Source: CAD feature listing. Evaluate the final solid. Frame: model axes, mm. Face numbers are marked on the shaded views. A direction names the side the tool comes from. Round coordinates to 2 decimals unless told otherwise and drop trailing zeros. Order: outer loops, then holes, each group sorted by start corner. A loop starts at its lowest first (then second) coordinate and runs counter-clockwise, first axis right, second up. Notation, with made-up numbers: (-7.75, -2) - (23.25, -2) arc R19 ccw to (23.25, 3) - close; hole circle Ø3 at (83, 14). An arc over 180 degrees is marked (long way). Return JSON: item names as keys, results as strings. Group by question number.
1) Ray query, line 1 (X direction, y = -2, z = 8.1); line 2 (X direction, y = -6.5, z = 7.4); line 3 (Y direction, x = 8, z = 7.75). Return the intervals inside material, ascending. Write a range as from..to.
2) Mould query, pull axis Z, two halves, no side actions, for the marked faces 1, 2 and 3. Classes: pulls with the +Z half, pulls with the -Z half, needs draft (parallel to the pull), parting line crosses it, or undercut.
3) Section B-B, the plane x = 0. Return loops of the section in (y, z), plus the area to 3 significant figures.
4) Section A-A, the plane y = 0. Return loops of the section in (x, z).
5) Access query for the marked faces 4, 5 and 6. Directions: +Z, -Z, +X, -X, +Y, -Y. A direction counts if a zero-diameter tool reaches every point of the face in a straight line with its end or side. Return the directions, or none.
6) Contact query for flat-ended pins moving along their axis: P1, Ø1, axis at x = -13, z = 7.5, coming from the -Y side; P2, Ø0.6, axis at x = 17.5, z = 7.5, coming from the -Y side; P3, Ø1.3, axis at y = 0, z = 7, coming from the +X side; P4, Ø13, axis at x = -7.5, y = -3.5, coming from the +Z side. Output: stop coordinate, or through.
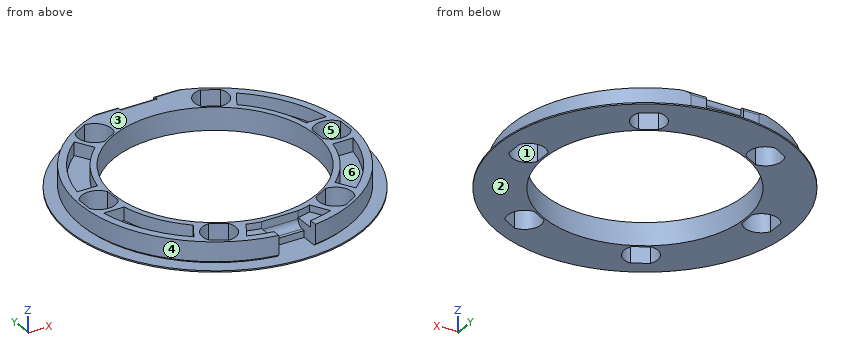
```python
from build123d import *

# Parameters (mm, degrees)
POCKET_DEPTH         = 128.037431
POLARPATTERN_COUNT   = 6
POCKET004_DEPTH      = 1.001
POCKET005_DEPTH      = 2.001
POCKET006_DEPTH      = 22.001
POCKET006_DEPTH_BACK = -22.001
POCKET007_DEPTH      = 2.75


with BuildPart() as part:
    # Sketch → Revolution (revolve)
    with BuildSketch(Plane.XZ):
        Polygon((19.85, 5.5), (22, 5.5), (22, 5.3), (15.1, 5.3), (15.1, 8.7), (20.15, 8.7), (20.15, 5.8), align=None)
    revolve(axis=Axis((0, 0, 0), (0, 0, 1)))

    # Sketch001 → Pocket (cut, through all)
    with BuildSketch(Plane.XY.offset(5.3)):
        with BuildLine():
            ThreePointArc((-15.35, 1.275735), (-17.5, 2.5), (-19.65, 1.275735))
            Line((-19.65, 1.275735), (-19.65, -1.275735))
            ThreePointArc((-19.65, -1.275735), (-17.5, -2.5), (-15.35, -1.275735))
            Line((-15.35, -1.275735), (-15.35, 1.275735))
        make_face()
    pocket = extrude(amount=POCKET_DEPTH, mode=Mode.SUBTRACT)

    # PolarPattern: Pocket ×6 about axis
    polarpattern_axis = Axis((0, 0, 0), (0, 0, 1))
    for i in range(1, POLARPATTERN_COUNT):
        add(pocket.rotate(polarpattern_axis, i * 360 / POLARPATTERN_COUNT), mode=Mode.SUBTRACT)

    # Sketch005 → Pocket004 (cut, through all)
    with BuildSketch(Plane.XY.offset(7.7)):
        with BuildLine():
            ThreePointArc((-4.775159, -15.270817), (0, -16), (4.775159, -15.270817))
            Line((4.775159, -15.270817), (6.306336, -17.922894))
            ThreePointArc((-6.306336, -17.922894), (0, -19), (6.306336, -17.922894))
            Line((-6.306336, -17.922894), (-4.775159, -15.270817))
        make_face()
    extrude(amount=POCKET004_DEPTH, mode=Mode.SUBTRACT)

    # Sketch006 → Pocket005 (cut, through all)
    with BuildSketch(Plane.XY.offset(6.7)):
        with BuildLine():
            ThreePointArc((-10.647805, 11.942539), (-13.856406, 8), (-15.666445, 3.25))
            Line((-15.666445, 3.25), (-18.719976, 3.25))
            ThreePointArc((-12.174571, 14.586975), (-16.454483, 9.5), (-18.719976, 3.25))
            Line((-12.174571, 14.586975), (-10.647805, 11.942539))
        make_face()
        with BuildLine():
            ThreePointArc((-15.666445, -3.25), (-13.856406, -8), (-10.647805, -11.942539))
            Line((-12.174571, -14.586975), (-10.647805, -11.942539))
            ThreePointArc((-18.719976, -3.25), (-16.454483, -9.5), (-12.174571, -14.586975))
            Line((-18.719976, -3.25), (-15.666445, -3.25))
        make_face()
        with BuildLine():
            ThreePointArc((10.647805, -11.942539), (13.856406, -8), (15.666445, -3.25))
            Line((15.666445, -3.25), (18.719976, -3.25))
            ThreePointArc((12.174571, -14.586975), (16.454483, -9.5), (18.719976, -3.25))
            Line((10.647805, -11.942539), (12.174571, -14.586975))
        make_face()
        with BuildLine():
            ThreePointArc((18.719976, 3.25), (16.454483, 9.5), (12.174571, 14.586975))
            Line((10.647805, 11.942539), (12.174571, 14.586975))
            ThreePointArc((15.666445, 3.25), (13.856406, 8), (10.647805, 11.942539))
            Line((15.666445, 3.25), (18.719976, 3.25))
        make_face()
    extrude(amount=POCKET005_DEPTH, mode=Mode.SUBTRACT)

    # Sketch008 → Pocket006 (cut, two sides)
    with BuildSketch(Plane.YZ) as pocket006_sk:
        with BuildLine():
            Line((19, 10), (19, 8.7))
            ThreePointArc((19.5, 8.2), (19.353553, 8.553553), (19, 8.7))
            Line((19.5, 8.2), (19.5, 5.5))
            Line((20.5, 5.5), (19.5, 5.5))
            Line((20.5, 10), (20.5, 5.5))
            Line((19, 10), (20.5, 10))
        make_face()
    extrude(amount=-POCKET006_DEPTH, mode=Mode.SUBTRACT)
    extrude(pocket006_sk.sketch, amount=-POCKET006_DEPTH_BACK, mode=Mode.SUBTRACT)

    # Sketch004 → Pocket007 (cut, symmetric)
    with BuildSketch(Plane.YZ):
        with BuildLine():
            Line((21, 11), (18.5, 11))
            Line((18.5, 11), (18.5, 8.7))
            ThreePointArc((18.722171, 7.752071), (18.986808, 8.314096), (18.5, 8.7))
            ThreePointArc((18.722171, 7.752071), (18.09345, 6.416824), (19.25, 5.5))
            Line((19.25, 5.5), (21, 5.5))
            Line((21, 5.5), (21, 11))
        make_face()
        with BuildLine():
            Line((-20.75, 11), (-20.75, 5.5))
            Line((-20.75, 5.5), (-19, 5.5))
            Line((-19, 5.5), (-17.25, 5.5))
            Line((-17.25, 5.5), (-17.25, 6.5))
            Line((-17.25, 6.5), (-16.75, 6.5))
            ThreePointArc((-16.75, 6.5), (-16.042893, 6.792893), (-15.75, 7.5))
            Line((-15.75, 7.5), (-15.75, 11))
            Line((-20.75, 11), (-15.75, 11))
        make_face()
    extrude(amount=POCKET007_DEPTH, both=True, mode=Mode.SUBTRACT)


solid = part.part
```
Geometry check:
{
 "1": {"line 1": "-20.05..-19, -16..-14.97, 14.97..16, 19..20.05", "line 2": "-19.07..-17.85, -14.62..-13.63, 13.63..14.62, 17.85..19.07", "line 3": "-18.49..-17.54, -13.11..-12.81, 12.81..13.11, 17.54..18.49"},
 "2": {"face 1": "needs draft", "face 2": "pulls with the -Z half", "face 3": "pulls with the +Z half"},
 "3": {"outline": "(-22, 5.3) - (-15.1, 5.3) - (-15.1, 8.7) - (-15.75, 8.7) - (-15.75, 7.5) arc R1 cw to (-16.75, 6.5) - (-17.25, 6.5) - (-17.25, 5.5) - (-22, 5.5) - close; (15.1, 5.3) - (22, 5.3) - (22, 5.5) - (19.25, 5.5) arc R1.19 cw to (18.72, 7.75) arc R0.5 ccw to (18.5, 8.7) - (15.1, 8.7) - close", "area": "17.3 mm2"},
 "4": {"outline": "(-22, 5.3) - (-19.65, 5.3) - (-19.65, 8.7) - (-20.15, 8.7) - (-20.15, 5.8) - (-19.85, 5.5) - (-22, 5.5) - close; (-15.35, 5.3) - (-15.1, 5.3) - (-15.1, 8.7) - (-15.35, 8.7) - close; (15.1, 5.3) - (15.35, 5.3) - (15.35, 8.7) - (15.1, 8.7) - close; (19.65, 5.3) - (22, 5.3) - (22, 5.5) - (19.85, 5.5) - (20.15, 5.8) - (20.15, 8.7) - (19.65, 8.7) - close"},
 "5": {"face 4": "+Z, -X", "face 5": "+Z, -Z", "face 6": "+Z"},
 "6": {"P1": "y = -15.8", "P2": "y = -10.5", "P3": "x = 20.15", "P4": "through"}
}
